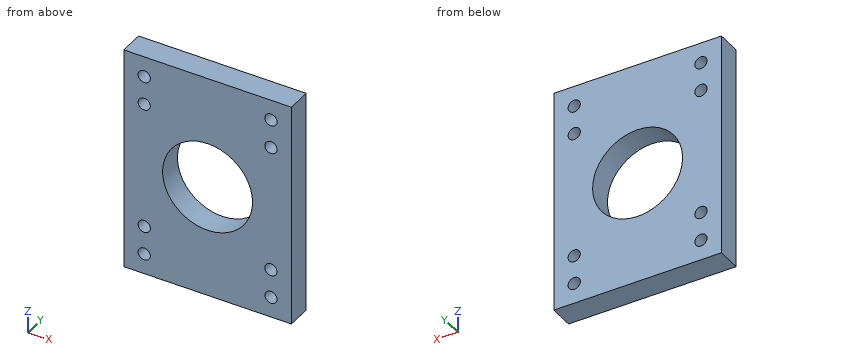
from build123d import *

# Parameters (mm, degrees)
F0_W     = 41
F0_H     = 55
F0_R     = 1.5
F0_R_2   = 11
F1_DEPTH = 6


with BuildPart() as f1:
    # F0 (on Front) → F1 (new body)
    with BuildSketch(Plane.XZ):
        Rectangle(F0_W, F0_H)
        with Locations((-15.5, -22.5)):
            Circle(F0_R, mode=Mode.SUBTRACT)
        with Locations((-15.5, -15.5)):
            Circle(F0_R, mode=Mode.SUBTRACT)
        with Locations((15.5, -22.5)):
            Circle(F0_R, mode=Mode.SUBTRACT)
        with Locations((15.5, -15.5)):
            Circle(F0_R, mode=Mode.SUBTRACT)
        with Locations((-15.5, 15.5)):
            Circle(F0_R, mode=Mode.SUBTRACT)
        with Locations((-15.5, 22.5)):
            Circle(F0_R, mode=Mode.SUBTRACT)
        Circle(F0_R_2, mode=Mode.SUBTRACT)
        with Locations((15.5, 15.5)):
            Circle(F0_R, mode=Mode.SUBTRACT)
        with Locations((15.5, 22.5)):
            Circle(F0_R, mode=Mode.SUBTRACT)
    extrude(amount=F1_DEPTH)


solid = f1.part
Model file for the job. Use its own axes, mm. Coordinates: 2 decimals unless noted, no trailing zeros. Write each loop counter-clockwise with the first axis right and the second up, starting at its lowest first coordinate (ties: lowest second). Pieces come first, ordered by that corner, then holes. Notation, with made-up numbers: (-39.5, -7) - (7.5, -7) arc R21 cw to (7.5, 5) - close; hole circle Ø1 at (-7, -7.75). An arc over 180 degrees is marked (long way). Write each question's results on one line, items separated by ' | '. Start each with the question number.
1) Cut at B-B (z = -22.5). Write the cut outline in (x, y).
2) Flat gauge pins, fed straight in: P1, Ø2.5, axis at x = 15.5, z = -22.5, coming from the +Y side; P2, Ø4, axis at x = -15.5, z = -15.5, coming from the +Y side. Where does each tip first touch, or does it go through?
3) Cut at D-D (x = 0). Write the cut outline in (y, z), then the cut area to 3 significant figures.
4) Cut at C-C (x = -15.5). Write the cut outline in (y, z).
5) Probe line 1 along Z through (x, y) = (15.5, -4.35); line 2 along X through (y, z) = (-3.95, 16); line 3 along Z through (x, y) = (-4.5, -5.4). List the from-to ranges inside material, lowest first. Write a range as from..to.
6) Cut at A-A (z = 0). Write the cut outline in (x, y).
Returned:
1) outline: (-20.5, -6) - (-17, -6) - (-17, 0) - (-20.5, 0) - close; (-14, -6) - (14, -6) - (14, 0) - (-14, 0) - close; (17, -6) - (20.5, -6) - (20.5, 0) - (17, 0) - close
2) P1: through | P2: y = 0
3) outline: (-6, -27.5) - (0, -27.5) - (0, -11) - (-6, -11) - close; (-6, 11) - (0, 11) - (0, 27.5) - (-6, 27.5) - close | area: 198 mm^2
4) outline: (-6, -27.5) - (0, -27.5) - (0, -24) - (-6, -24) - close; (-6, -21) - (0, -21) - (0, -17) - (-6, -17) - close; (-6, -14) - (0, -14) - (0, 14) - (-6, 14) - close; (-6, 17) - (0, 17) - (0, 21) - (-6, 21) - close; (-6, 24) - (0, 24) - (0, 27.5) - (-6, 27.5) - close
5) line 1: -27.5..-24, -21..-17, -14..14, 17..21, 24..27.5 | line 2: -20.5..-16.91, -14.09..14.09, 16.91..20.5 | line 3: -27.5..-10.04, 10.04..27.5
6) outline: (-20.5, -6) - (-11, -6) - (-11, 0) - (-20.5, 0) - close; (11, -6) - (20.5, -6) - (20.5, 0) - (11, 0) - close
